from build123d import *

# Parameters (mm, degrees)
MODEL_R             = 3.25
MODEL_W             = 6.88
MODEL_H             = 15
BOSS_EXTRUDE1_DEPTH = 6.6


with BuildPart() as part:
    # Model → Boss-Extrude1 (new body)
    with BuildSketch(Plane.XY):
        with BuildLine():
            Line((39.57, 15.5), (39.57, 11.5))
            ThreePointArc((39.57, 11.5), (39.423553391, 11.146446609), (39.07, 11))
            Line((39.07, 11), (37.985, 11))
            ThreePointArc((37.985, 11), (37.631446609, 10.853553391), (37.485, 10.5))
            Line((37.485, 10.5), (37.485, 0))
            Line((37.485, 0), (71.42, 0))
            Line((71.42, 0), (71.42, 59))
            ThreePointArc((71.42, 59), (70.687766953, 60.767766953), (68.92, 61.5))
            Line((68.92, 61.5), (58.92, 61.5))
            ThreePointArc((58.92, 61.5), (57.152233047, 60.767766953), (56.42, 59))
            Line((56.42, 59), (56.42, 55))
            Line((56.42, 55), (37.485, 55))
            Line((37.485, 55), (37.485, 44))
            Line((37.485, 44), (39.07, 44))
            ThreePointArc((39.07, 44), (39.423553391, 43.853553391), (39.57, 43.5))
            Line((39.57, 43.5), (39.57, 39.5))
            ThreePointArc((39.57, 39.5), (39.423553391, 39.146446609), (39.07, 39))
            Line((39.07, 39), (37.485, 39))
            Line((37.485, 39), (37.485, 34.5))
            ThreePointArc((37.485, 34.5), (37.338553391, 34.146446609), (36.985, 34))
            Line((36.985, 34), (34.435, 34))
            ThreePointArc((34.435, 34), (34.081446609, 34.146446609), (33.935, 34.5))
            Line((33.935, 34.5), (33.935, 39))
            Line((33.935, 39), (32.35, 39))
            ThreePointArc((32.35, 39), (31.996446609, 39.146446609), (31.85, 39.5))
            Line((31.85, 39.5), (31.85, 43.5))
            ThreePointArc((31.85, 43.5), (31.996446609, 43.853553391), (32.35, 44))
            Line((32.35, 44), (33.935, 44))
            Line((33.935, 44), (33.935, 55))
            Line((33.935, 55), (0, 55))
            Line((0, 55), (0, -4))
            ThreePointArc((0, -4), (0.732233047, -5.767766953), (2.5, -6.5))
            Line((2.5, -6.5), (12.5, -6.5))
            ThreePointArc((12.5, -6.5), (14.267766953, -5.767766953), (15, -4))
            Line((15, -4), (15, 0))
            Line((15, 0), (33.935, 0))
            Line((33.935, 0), (33.935, 10.5))
            ThreePointArc((33.935, 10.5), (33.788553391, 10.853553391), (33.435, 11))
            Line((33.435, 11), (32.35, 11))
            ThreePointArc((32.35, 11), (31.996446609, 11.146446609), (31.85, 11.5))
            Line((31.85, 11.5), (31.85, 15.5))
            ThreePointArc((31.85, 15.5), (31.996446609, 15.853553391), (32.35, 16))
            Line((32.35, 16), (33.935, 16))
            Line((33.935, 16), (33.935, 20.5))
            ThreePointArc((33.935, 20.5), (34.081446609, 20.853553391), (34.435, 21))
            Line((34.435, 21), (36.985, 21))
            ThreePointArc((36.985, 21), (37.338553391, 20.853553391), (37.485, 20.5))
            Line((37.485, 20.5), (37.485, 16))
            Line((37.485, 16), (39.07, 16))
            ThreePointArc((39.07, 16), (39.423553391, 15.853553391), (39.57, 15.5))
        make_face()
        with Locations((23.174807377, 12.7)):
            Circle(MODEL_R, mode=Mode.SUBTRACT)
        with Locations((23.174807377, 42.3)):
            Circle(MODEL_R, mode=Mode.SUBTRACT)
        with Locations((48.245192623, 12.7)):
            Circle(MODEL_R, mode=Mode.SUBTRACT)
        with Locations((48.245192623, 42.3)):
            Circle(MODEL_R, mode=Mode.SUBTRACT)
        with Locations((7.78, 27.5)):
            Rectangle(MODEL_W, MODEL_H, mode=Mode.SUBTRACT)
        with Locations((63.64, 27.5)):
            Rectangle(MODEL_W, MODEL_H, mode=Mode.SUBTRACT)
    extrude(amount=BOSS_EXTRUDE1_DEPTH)


solid = part.part
Read the model definition and answer for the solid it produces. Units are mm, in the model's axes. A direction names the side the tool comes from. Round coordinates to 2 decimals unless told otherwise and drop trailing zeros. Loops run counter-clockwise (first coordinate to the right, second up) from the corner with the lowest first, then second, coordinate; pieces in that order, holes last. Notation, with made-up numbers: (85.5, 80) - (116.5, 80) arc R20 ccw to (116.5, 93) - close; hole circle Ø9 at (74, 66). An arc over 180 degrees is marked (long way). One line per question, with ' | ' between items. Start each with the question number.
Q1. Section C-C on z = 4 is taken. Count the separate pieces of the cut face and the enclosed holes in it, plus the area to 3 significant figures.
Q2. Find the intervals of material crossed by L1, parallel to Y at x = 48, z = 2.5; L2, parallel to X at y = 30.5, z = 3.75; L3, parallel to X at y = 3.5, z = 6 (3 decimals), in increasing order.
Q3. Section A-A on y = 12.7 is taken. Give the vertices of the cut face in (x, z), plus the area to 3 significant figures.
Q4. For faces 4 (the flat face through (33, 39, 3)), 5 (the flat face through (7, -6.5, 3)), 6 (the flat face through (37.485, 18, 3)), 7 (the flat face through (36, 34, 3)), 8 (the flat face through (54, 0, 3)), determine the directions among +Z, -Z, +X, -X, +Y, -Y from which every point of the face is accessible in a straight line to the end or side of a thin tool.
Q5. Section B-B on x = 10 is taken. Give the vertices of the cut face in (y, z).
Q6. For a pull along X with two mould halves and no side action, classify faces 1 (the cylindrical face through (70.707, 60.748, 3.254)), 2 (the flat face through (47, 55, 3)), 3 (the flat face through (37.485, 37, 3)) as +X half, -X half, draft (parallel to the pull), parting line (faces both ways), or undercut.
Q7. Section D-D on x = 41 is taken. Give the vertices of the cut face in (y, z).
Q8. Flat-ended cylindrical pins translate along their axes: pin 1 (3.5 mm diameter, centred on x = 12.5, z = 3, fed in from +Y); pin 2 (1.5 mm diameter, centred on x = 19.5, z = 5.5, fed in from -Y). Find the tip coordinate at first contact, or state that the pin passes through.
Established:
1) separate pieces: 1 | enclosed holes: 6 | area: 3,590 mm²
2) L1: 0 to 9.46, 15.94 to 39.06, 45.54 to 55 | L2: 0 to 4.34, 11.22 to 60.2, 67.08 to 71.42 | L3: 0 to 33.935, 37.485 to 71.42
3) outline: (0, 0) - (19.92, 0) - (19.92, 6.6) - (0, 6.6) - close; (26.42, 0) - (31.85, 0) - (31.85, 6.6) - (26.42, 6.6) - close; (39.57, 0) - (45, 0) - (45, 6.6) - (39.57, 6.6) - close; (51.5, 0) - (71.42, 0) - (71.42, 6.6) - (51.5, 6.6) - close | area: 335 mm²
4) face 4: +Z, -Z | face 5: +Z, -Z, +X, -X, -Y | face 6: +Z, -Z, -Y | face 7: +Z, -Z, +Y | face 8: +Z, -Z, +X, -Y
5) outline: (-6.5, 0) - (20, 0) - (20, 6.6) - (-6.5, 6.6) - close; (35, 0) - (55, 0) - (55, 6.6) - (35, 6.6) - close
6) face 1: +X half | face 2: draft | face 3: undercut
7) outline: (0, 0) - (55, 0) - (55, 6.6) - (0, 6.6) - close
8) pin 1: y = 55 | pin 2: y = 0
